Verification items for the finished model (mm, model axes). Give positions to 0.01 mm unless a question says otherwise; leave off trailing zeros. Write each loop counter-clockwise with the first axis right and the second up, starting at its lowest first coordinate (ties: lowest second). Pieces come first, ordered by that corner, then holes. Notation, with made-up numbers: M 43.5,7.25 L 47.5,7.25 A18 cw 47.5,15.25 Z; hole C 19.5,52.5 d10. An arc over 180 degrees is marked long. Answer as a JSON object with one key per item and string values.
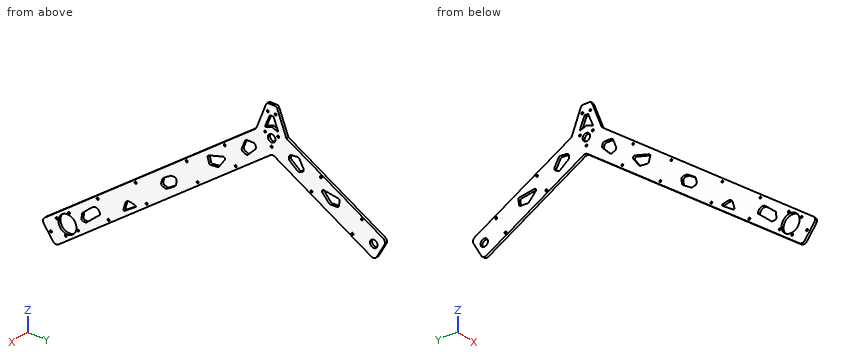
```python
from build123d import *

# Parameters (mm, degrees)
SKETCH3_R                           = 4.765
SKETCH3_R_2                         = 11.5
SKETCH3_R_3                         = 1.25
BOSS_ROCKER_BASE_DEPTH              = 3.18
SKETCH4_R                           = 1.25
CUT_MOTOR_HOLES_SHAFT_SUPPORT_DEPTH = 3.18
SKETCH5_R                           = 1.25
CUT_SUPPORT_HOLES_DEPTH             = 3.18
CUT_LIGHTENING_HOLES_DEPTH          = 3.18


with BuildPart() as part:
    # Sketch3 → Boss-rocker base (new body)
    with BuildSketch(Plane.YZ):
        with BuildLine():
            Line((-19.740098585, 194.326279503), (-289.03382674, -2.652716496))
            ThreePointArc((-289.03382674, -2.652716496), (-291.022843538, -5.922039532), (-290.117530314, -9.640247287))
            Line((-290.117530314, -9.640247287), (-278.309875879, -25.782716018))
            ThreePointArc((-278.309875879, -25.782716018), (-275.040552842, -27.771732816), (-271.322345088, -26.866419592))
            Line((-271.322345088, -26.866419592), (-1.602441241, 170.424309102))
            ThreePointArc((-1.602441241, 170.424309102), (1.066332673, 171.380668673), (3.826130086, 170.732211983))
            Line((3.826130086, 170.732211983), (126.91354691, 100.548260636))
            ThreePointArc((126.91354691, 100.548260636), (130.710275653, 100.069186741), (133.733724692, 102.415122982))
            Line((133.733724692, 102.415122982), (143.640355564, 119.789203239))
            ThreePointArc((143.640355564, 119.789203239), (144.119429459, 123.585931982), (141.773493218, 126.609381021))
            Line((141.773493218, 126.609381021), (18.794188293, 196.731687397))
            Line((18.794188293, 196.731687397), (7.025536002, 226.658847865))
            ThreePointArc((7.025536002, 226.658847865), (5.922779586, 228.040238472), (4.233648495, 228.560957093))
            Line((4.233648495, 228.560957093), (-4.233648495, 228.560957093))
            ThreePointArc((-4.233648495, 228.560957093), (-5.922779586, 228.040238472), (-7.025536002, 226.658847865))
            Line((-7.025536002, 226.658847865), (-19.740098585, 194.326279503))
        make_face()
        with Locations((0, 190.180957093)):
            Circle(SKETCH3_R, mode=Mode.SUBTRACT)
        with Locations((-260, 0)):
            Circle(SKETCH3_R_2, mode=Mode.SUBTRACT)
        with Locations((130, 116.055478547)):
            Circle(SKETCH3_R, mode=Mode.SUBTRACT)
        with Locations((-5, 219.130957093)):
            Circle(SKETCH3_R_3, mode=Mode.SUBTRACT)
        with Locations((5, 219.130957093)):
            Circle(SKETCH3_R_3, mode=Mode.SUBTRACT)
    extrude(amount=BOSS_ROCKER_BASE_DEPTH)

    # Sketch4 → Cut-motor holes + shaft support (cut)
    with BuildSketch(Plane.YZ):
        with Locations((0, 180.656752709)):
            Circle(SKETCH4_R)
        with Locations((-8.24, 194.928851363)):
            Circle(SKETCH4_R)
        with Locations((8.24, 194.928851363)):
            Circle(SKETCH4_R)
        with Locations((-273.836126141, 2.145136678)):
            Circle(SKETCH4_R)
        with Locations((-257.855082097, 13.834714568)):
            Circle(SKETCH4_R)
        with Locations((-262.144917759, -13.834714591)):
            Circle(SKETCH4_R)
        with Locations((-246.163873715, -2.1451367)):
            Circle(SKETCH4_R)
    extrude(amount=CUT_MOTOR_HOLES_SHAFT_SUPPORT_DEPTH, mode=Mode.SUBTRACT)

    # Sketch5 → Cut-support holes (cut)
    with BuildSketch(Plane.YZ):
        with Locations((-173.097097557, 78.211050768)):
            Circle(SKETCH5_R)
        with Locations((-159.140450015, 59.130652728)):
            Circle(SKETCH5_R)
        with Locations((-94.167013372, 106.656461829)):
            Circle(SKETCH5_R)
        with Locations((-108.123660914, 125.73685987)):
            Circle(SKETCH5_R)
        with Locations((-221.524503751, 42.788087462)):
            Circle(SKETCH5_R)
        with Locations((-207.567856209, 23.707689422)):
            Circle(SKETCH5_R)
        with Locations((-45.739607178, 142.079425135)):
            Circle(SKETCH5_R)
        with Locations((-59.69625472, 161.159823175)):
            Circle(SKETCH5_R)
        with Locations((103.007538851, 117.839995969)):
            Circle(SKETCH5_R)
        with Locations((114.717176541, 138.376158833)):
            Circle(SKETCH5_R)
        with Locations((62.594935771, 168.096051448)):
            Circle(SKETCH5_R)
        with Locations((50.885298081, 147.559888585)):
            Circle(SKETCH5_R)
        with Locations((-280.985209351, -15.349950766)):
            Circle(SKETCH5_R)
    extrude(amount=CUT_SUPPORT_HOLES_DEPTH, mode=Mode.SUBTRACT)

    # Sketch6 → Cut-lightening holes (cut)
    with BuildSketch(Plane.YZ):
        with BuildLine():
            Line((-79.983471427, 142.368791683), (-61.979782767, 147.316428458))
            ThreePointArc((-61.979782767, 147.316428458), (-59.811067724, 146.534457497), (-59.819745898, 144.229088067))
            Line((-59.819745898, 144.229088067), (-67.122963599, 133.95613022))
            ThreePointArc((-67.122963599, 133.95613022), (-67.760393878, 133.378682327), (-68.581402, 133.122344477))
            Line((-68.581402, 133.122344477), (-77.604831251, 132.34516891))
            ThreePointArc((-77.604831251, 132.34516891), (-78.919471752, 132.69660063), (-79.704956379, 133.807815192))
            Line((-79.704956379, 133.807815192), (-81.381998087, 139.910311831))
            ThreePointArc((-81.381998087, 139.910311831), (-81.191902606, 141.429196112), (-79.983471427, 142.368791683))
        make_face()
        with BuildLine():
            Line((-23.474916203, 177.031971532), (-31.234891161, 177.031971532))
            ThreePointArc((-31.234891161, 177.031971532), (-32.91387852, 176.518133523), (-34.017714198, 175.152639164))
            Line((-34.017714198, 175.152639164), (-37.880265406, 165.561216901))
            ThreePointArc((-37.880265406, 165.561216901), (-37.857627092, 163.26522791), (-36.218110002, 161.657726231))
            Line((-36.218110002, 161.657726231), (-33.122502329, 160.411097438))
            ThreePointArc((-33.122502329, 160.411097438), (-31.392547815, 160.256443753), (-29.866816812, 161.086386695))
            Line((-29.866816812, 161.086386695), (-20.893300564, 170.176925526))
            ThreePointArc((-20.893300564, 170.176925526), (-20.132536099, 171.500594144), (-20.121734598, 173.027271748))
            Line((-20.121734598, 173.027271748), (-20.568332353, 174.774783973))
            ThreePointArc((-20.568332353, 174.774783973), (-21.634866927, 176.401405781), (-23.474916203, 177.031971532))
        make_face()
        with BuildLine():
            Line((-123.842513182, 102.258163939), (-127.383477271, 102.258163939))
            ThreePointArc((-127.383477271, 102.258163939), (-128.217930269, 102.139776022), (-128.986523832, 101.793956069))
            Line((-128.986523832, 101.793956069), (-137.87452461, 96.175246667))
            ThreePointArc((-137.87452461, 96.175246667), (-138.681600876, 95.425877769), (-139.163866001, 94.435753436))
            Line((-139.163866001, 94.435753436), (-140.452603638, 89.754685534))
            ThreePointArc((-140.452603638, 89.754685534), (-140.168511172, 87.476227852), (-138.356514585, 86.065998684))
            Line((-138.356514585, 86.065998684), (-135.427175254, 85.259526758))
            ThreePointArc((-135.427175254, 85.259526758), (-134.189854142, 85.184508534), (-133.027829794, 85.61612258))
            Line((-133.027829794, 85.61612258), (-123.19292846, 91.833432183))
            ThreePointArc((-123.19292846, 91.833432183), (-122.319685125, 92.675710701), (-121.851449189, 93.794970338))
            Line((-121.851449189, 93.794970338), (-120.89798735, 98.683909964))
            ThreePointArc((-120.89798735, 98.683909964), (-121.527047578, 101.165680397), (-123.842513182, 102.258163939))
        make_face()
        with BuildLine():
            Line((-173.179518759, 50.529751316), (-187.062617136, 41.348992712))
            ThreePointArc((-187.062617136, 41.348992712), (-188.206182034, 41.377149334), (-188.575130176, 42.459928509))
            Line((-188.575130176, 42.459928509), (-186.300929891, 50.354284082))
            ThreePointArc((-186.300929891, 50.354284082), (-184.055505641, 53.265590831), (-180.426317386, 53.854343461))
            Line((-180.426317386, 53.854343461), (-173.517109299, 52.340698989))
            ThreePointArc((-173.517109299, 52.340698989), (-172.74804587, 51.547125046), (-173.179518759, 50.529751316))
        make_face()
        with BuildLine():
            Line((-227.536912906, 31.443521835), (-240.812092581, 20.074883922))
            ThreePointArc((-240.812092581, 20.074883922), (-241.294394217, 19.461411125), (-241.505216951, 18.71006732))
            Line((-241.505216951, 18.71006732), (-241.969357294, 12.71062362))
            ThreePointArc((-241.969357294, 12.71062362), (-241.494399162, 11.255439603), (-240.129582559, 10.562315233))
            Line((-240.129582559, 10.562315233), (-237.156438151, 10.332301196))
            ThreePointArc((-237.156438151, 10.332301196), (-236.381608619, 10.425053213), (-235.701254134, 10.807259329))
            Line((-235.701254134, 10.807259329), (-219.133655325, 24.995468947))
            ThreePointArc((-219.133655325, 24.995468947), (-218.552793599, 25.837124808), (-218.463915883, 26.855891554))
            ThreePointArc((-218.463915883, 26.855891554), (-221.531743706, 31.287956059), (-226.896432107, 31.812247659))
            ThreePointArc((-226.896432107, 31.812247659), (-227.233851743, 31.657725269), (-227.536912906, 31.443521835))
        make_face()
        with BuildLine():
            Line((85.568117513, 143.181930885), (86.544369033, 149.434919538))
            ThreePointArc((86.544369033, 149.434919538), (86.183746182, 150.922567652), (84.87682125, 151.719494858))
            Line((84.87682125, 151.719494858), (66.429148509, 154.599648582))
            ThreePointArc((66.429148509, 154.599648582), (64.362763101, 153.577467158), (64.632063287, 151.28786437))
            Line((64.632063287, 151.28786437), (73.050048081, 141.906596667))
            ThreePointArc((73.050048081, 141.906596667), (73.74868466, 141.404929088), (74.593412473, 141.243070035))
            Line((74.593412473, 141.243070035), (83.646848899, 141.491195361))
            ThreePointArc((83.646848899, 141.491195361), (84.913320183, 141.989025039), (85.568117513, 143.181930885))
        make_face()
        with BuildLine():
            Line((21.93232317, 175.41253387), (22.178458249, 177.199337176))
            ThreePointArc((22.178458249, 177.199337176), (23.054223795, 178.936124213), (24.811171332, 179.770707856))
            Line((24.811171332, 179.770707856), (32.521378103, 180.648160365))
            ThreePointArc((32.521378103, 180.648160365), (34.247699157, 180.327467884), (35.498857547, 179.095546323))
            Line((35.498857547, 179.095546323), (40.421178328, 170.0023928))
            ThreePointArc((40.421178328, 170.0023928), (40.658302188, 167.718569205), (39.211066927, 165.935990164))
            Line((39.211066927, 165.935990164), (36.27627425, 164.347323378))
            ThreePointArc((36.27627425, 164.347323378), (34.574902041, 163.998048434), (32.965111147, 164.650147857))
            Line((32.965111147, 164.650147857), (23.021241192, 172.667712351))
            ThreePointArc((23.021241192, 172.667712351), (22.115683157, 173.896868902), (21.93232317, 175.41253387))
        make_face()
        with BuildLine():
            Line((1.921390016, 215.785081873), (-1.921390016, 215.785081873))
            ThreePointArc((-1.921390016, 215.785081873), (-2.199739759, 215.700438853), (-2.38384805, 215.475167556))
            Line((-2.38384805, 215.475167556), (-8.248888496, 201.206154542))
            ThreePointArc((-8.248888496, 201.206154542), (-8.149028051, 200.671797182), (-7.620562901, 200.544382574))
            Line((-7.620562901, 200.544382574), (-0.165867561, 203.165811621))
            ThreePointArc((-0.165867561, 203.165811621), (0, 203.194125335), (0.165867561, 203.165811621))
            Line((0.165867561, 203.165811621), (7.620562901, 200.544382574))
            ThreePointArc((7.620562901, 200.544382574), (8.149028051, 200.671797182), (8.248888496, 201.206154542))
            Line((8.248888496, 201.206154542), (2.38384805, 215.475167556))
            ThreePointArc((2.38384805, 215.475167556), (2.199739759, 215.700438853), (1.921390016, 215.785081873))
        make_face()
    extrude(amount=CUT_LIGHTENING_HOLES_DEPTH, mode=Mode.SUBTRACT)


solid = part.part
```
1) Section check C-C on y = -116.5. Record the boundary of the cut face in (x, z), and give its area (3 significant figures).
Completed:
{"outline": "M 0,86.38 L 3.18,86.38 L 3.18,123.55 L 0,123.55 Z", "area": "118 mm2"}
2) Section check A-A on y = 79. Record the boundary of the cut face in (x, z), and give its area (3 significant figures).
Completed:
{"outline": "M 0,127.87 L 3.18,127.87 L 3.18,141.36 L 0,141.36 Z; M 0,152.64 L 3.18,152.64 L 3.18,162.4 L 0,162.4 Z", "area": "74.0 mm2"}
3) Go/stop test with flat-tipped pins: pin 1 (1.5 mm diameter, centred on x = 2, y = -234.5, fed in from -Z); pin 2 (3 mm diameter, centred on y = -108.12, z = 125.74, fed in from +X); pin 3 (1.5 mm diameter, centred on x = 1, z = 122.5, fed in from -Y); pin 4 (1.6 mm diameter, centred on x = 2.5, y = -28, fed in from -Z). Record where each tip stops, or that it passes through.
Completed:
{"pin 1": "stops at z = -0.48", "pin 2": "stops at x = 3.18", "pin 3": "stops at y = -118.96", "pin 4": "stops at z = 150.53"}
4) Thickness scan on L1, parallel to Y at x = 0.65, z = 116; L2, parallel to Y at x = 2.3, z = 30; L3, parallel to Y at x = 0.2, z = 122. Record the ranges inside material, lowest first.
Completed:
{"L1": "y = -126.82 to -76.01, 99.81 to 125.24, 134.76 to 141.48", "L2": "y = -244.39 to -229.22, -219.97 to -193.58", "L3": "y = -118.62 to -67.8, 89.29 to 144.29"}
5) Section check B-B on x = 1.4. Count the separate pieces of the cut face and the enclosed holes in it, and give its area (3 significant figures).
Completed:
{"separate pieces": "1", "enclosed holes": "33", "area": "13,700 mm2"}
